Drawing for the job (mm, zero at the part's lowest x, y, z). A direction names the side the tool comes from. Round coordinates to 2 decimals unless told otherwise and drop trailing zeros. Order: outer loops, then holes, each group sorted by start corner. A loop starts at its lowest first (then second) coordinate and runs counter-clockwise, first axis right, second up. Notation, with made-up numbers: M 47.5,29.5 L 54.5,29.5 A24 ccw 54.5,51.5 Z; hole C 85,54.25 d1. An arc over 180 degrees is marked long. One line per item, written item: value. Start each with the question number.
Item 1: Tool access for the marked faces 3, 4 and 5: list every direction of +Z, -Z, +X, -X, +Y, -Y with a clear straight run to the whole face (end or side of a thin tool).
Item 2: Band-saw the part on C-C, the plane y = 5.5. Write the cut outline in (x, z), then the cut area to 3 significant figures.
Item 3: Band-saw the part on A-A, the plane x = 28.9. Write the cut outline in (y, z).
Item 4: Pin check, flat tips, straight feed: pin 1 (3 mm diameter, centred on x = 10.5, y = 2, fed in from -Z); pin 2 (1.5 mm diameter, centred on x = 11.5, y = 6, fed in from +Z); pin 3 (1.5 mm diameter, centred on x = 16, z = 1.5, fed in from +Y). Stop position of each tip, or through.
Item 5: Probe L1, parallel to X at y = 3.5, z = 0.7; L2, parallel to X at y = 4, z = 2.15; L3, parallel to Y at x = 29, z = 0.35 (1 decimal). List the from-to ranges inside material, lowest first.
Item 6: Band-saw the part on B-B, the plane z = 0.9. Write the cut outline in (x, y).
Item 7: Band-saw the part on D-D, the plane x = 16. Write the cut outline in (y, z), then the cut area to 3 significant figures.
Item 8: Two-plate mould, pull along X, no slides. Class the marked faces 1 and 2: +X half, -X half, draft (parallel to the pull), parting line (faces both ways), or undercut.
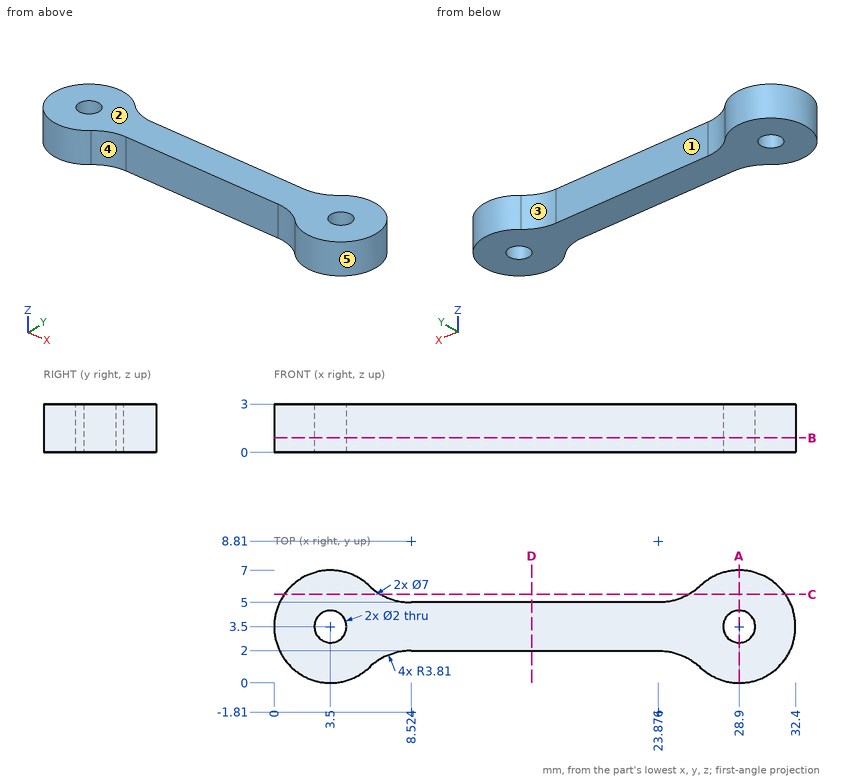
Output:
1. face 3: +Z, -Z, +Y
1. face 4: +Z, -Z, -Y
1. face 5: +Z, -Z
2. outline: M 0.63,0 L 6.64,0 L 6.64,3 L 0.63,3 Z; M 25.76,0 L 31.77,0 L 31.77,3 L 25.76,3 Z
2. area: 36.1 mm²
3. outline: M 0,0 L 2.5,0 L 2.5,3 L 0,3 Z; M 4.5,0 L 7,0 L 7,3 L 4.5,3 Z
4. pin 1: stops at z = 0
4. pin 2: passes through
4. pin 3: stops at y = 5
5. L1: x = 0 to 2.5, 4.5 to 27.9, 29.9 to 32.4
5. L2: x = 0.04 to 2.63, 4.37 to 28.03, 29.77 to 32.36
5. L3: y = 0 to 2.5, 4.5 to 7
6. outline: M 5.91,0.96 A3.81 cw 8.52,2 L 23.88,2 A3.81 cw 26.49,0.96 A3.5 ccw long 26.49,6.04 A3.81 cw 23.88,5 L 8.52,5 A3.81 cw 5.91,6.04 A3.5 ccw long Z; hole C 3.5,3.5 d2; hole C 28.9,3.5 d2
7. outline: M 2,0 L 5,0 L 5,3 L 2,3 Z
7. area: 9.00 mm²
8. face 1: undercut
8. face 2: draft
